from build123d import *

# Parameters (mm, degrees)
BOSS_EXTRUDE1_DEPTH = 50
CUT_EXTRUDE1_DEPTH  = 48
FILLET1_R           = 1


with BuildPart() as part:
    # Sketch1 → Boss-Extrude1 (new body)
    with BuildSketch(Plane.XY):
        with BuildLine():
            Line((25, 9), (-25, 9))
            ThreePointArc((-25, 9), (-26.414213562, 8.414213562), (-27, 7))
            Line((-27, 7), (-27, -7))
            ThreePointArc((-27, -7), (-26.414213562, -8.414213562), (-25, -9))
            Line((-25, -9), (25, -9))
            ThreePointArc((25, -9), (26.414213562, -8.414213562), (27, -7))
            Line((27, -7), (27, 7))
            ThreePointArc((27, 7), (26.414213562, 8.414213562), (25, 9))
        make_face()
    extrude(amount=BOSS_EXTRUDE1_DEPTH)

    # Sketch2 → Cut-Extrude1 (cut)
    with BuildSketch(Plane.XY.offset(50)):
        with BuildLine():
            Line((24, -7.5), (-24, -7.5))
            ThreePointArc((-24, -7.5), (-25.414213562, -6.914213562), (-26, -5.5))
            Line((-26, -5.5), (-26, 5.5))
            ThreePointArc((-26, 5.5), (-25.414213562, 6.914213562), (-24, 7.5))
            Line((-24, 7.5), (24, 7.5))
            ThreePointArc((24, 7.5), (25.414213562, 6.914213562), (26, 5.5))
            Line((26, 5.5), (26, -5.5))
            ThreePointArc((26, -5.5), (25.414213562, -6.914213562), (24, -7.5))
        make_face()
    extrude(amount=-CUT_EXTRUDE1_DEPTH, mode=Mode.SUBTRACT)

    # Fillet1
    fillet1_edges = [part.edges().sort_by_distance(p)[0] for p in [
        (0, -9, 0),
        (-26.414213562, -8.414213562, 0),
        (-27, 0, 0),
        (-26.414213562, 8.414213562, 0),
        (0, 9, 0),
        (26.414213562, 8.414213562, 0),
        (27, 0, 0),
        (26.414213562, -8.414213562, 0),
    ]]
    fillet(fillet1_edges, radius=FILLET1_R)


solid = part.part
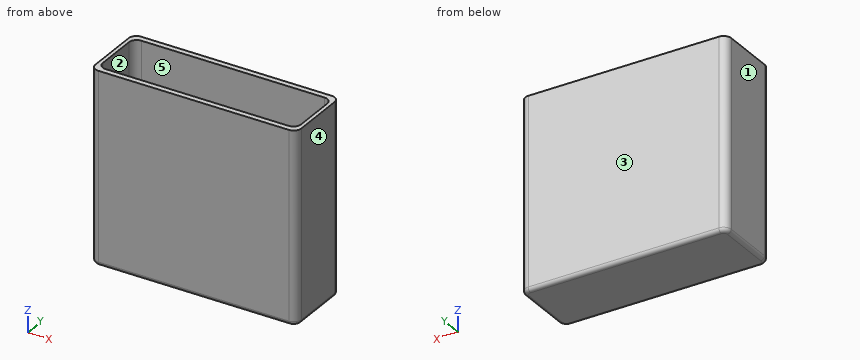
Can you work these out from the model? Positions are in its coordinate system, mm. Face numbers are marked on the shaded views. A direction names the side the tool comes from. Coordinates: 2 decimals unless noted, no trailing zeros. Write each loop counter-clockwise with the first axis right and the second up, starting at its lowest first coordinate (ties: lowest second). Pieces come first, ordered by that corner, then holes. Notation, with made-up numbers: (44.5, -9) -> (75.5, -9) arc R17 cw to (75.5, 21) -> close; hole circle Ø7 at (-9.5, 83.25). An arc over 180 degrees is marked (long way). Answer as CSV lines item,"result".
1) On a 3-axis mill with a long thin cutter (end or side, diameter ignored), from which of +Z, -Z, +X, -X, +Y, -Y can I reach the whole of each face in a straight line? I mean the marked faces 4 and 5. Say none if no direction works.
Check result:
face 4,"+Z, -Z, +X, +Y, -Y"
face 5,"+Z"
2) If we section it at C-C on y = 0.5: Please give me the cut outline in (x, z).
Check result:
outline,"(-27, 1) arc R1 ccw to (-26, 0) -> (26, 0) arc R1 ccw to (27, 1) -> (27, 50) -> (26, 50) -> (26, 2) -> (-26, 2) -> (-26, 50) -> (-27, 50) -> close"
3) If we mould it in two halves opening along X, with no side actions, what happens to the marked faces 1, 2 and 3? For each: +X half, -X half, draft (parallel to the pull), parting line (faces both ways), or undercut.
Check result:
face 1,"-X half"
face 2,"undercut"
face 3,"draft"
4) If I drill on line 1 (X direction, y = -4.5, z = 20); line 2 (Y direction, x = -9.5, z = 41); line 3 (Z direction, x = -17.5, y = -3.5), over which ranges is the centre line in solid material (lowest first)? Write a range as from..to.
Check result:
line 1,"-27..-26, 26..27"
line 2,"-9..-7.5, 7.5..9"
line 3,"0..2"
5) If we section it at B-B on x = 15.5: Please give me the cut outline in (y, z), then the cut area to 3 significant figures.
Check result:
outline,"(-9, 1) arc R1 ccw to (-8, 0) -> (8, 0) arc R1 ccw to (9, 1) -> (9, 50) -> (7.5, 50) -> (7.5, 2) -> (-7.5, 2) -> (-7.5, 50) -> (-9, 50) -> close"
area,"180 mm²"
6) If we section it at A-A on z = 38: Please give me the cut outline in (x, y), then the cut area to 3 significant figures.
Check result:
outline,"(-27, -7) arc R2 ccw to (-25, -9) -> (25, -9) arc R2 ccw to (27, -7) -> (27, 7) arc R2 ccw to (25, 9) -> (-25, 9) arc R2 ccw to (-27, 7) -> close; hole (-26, -5.5) arc R2 ccw to (-24, -7.5) -> (24, -7.5) arc R2 ccw to (26, -5.5) -> (26, 5.5) arc R2 ccw to (24, 7.5) -> (-24, 7.5) arc R2 ccw to (-26, 5.5) -> close"
area,"192 mm²"
